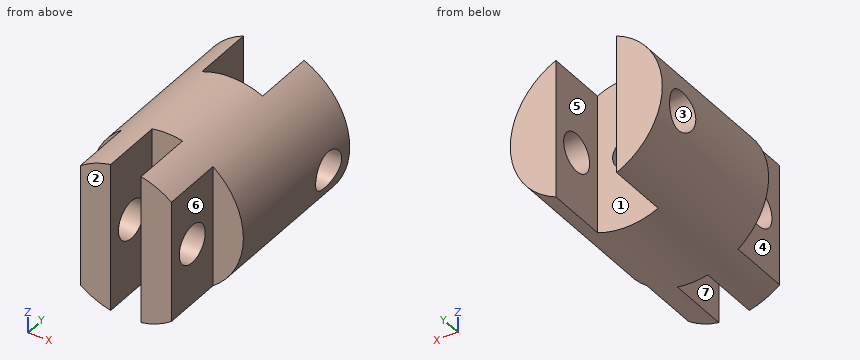
from build123d import *

# Parameters (mm, degrees)
SKETCH1_R               = 12.7
BOSS_EXTRUDE1_DEPTH     = 36.195
CUT_EXTRUDE1_START      = -10.16
CUT_EXTRUDE1_DEPTH      = 10.16
CUT_EXTRUDE2_DEPTH      = 10.16
CUT_EXTRUDE3_DEPTH      = 43.278794034
CUT_EXTRUDE3_DEPTH_BACK = 43.278794034
SKETCH4_R               = 3.175
SKETCH5_R               = 2.54
CUT_EXTRUDE4_DEPTH      = 32.629120053


with BuildPart() as part:
    # Sketch1 → Boss-Extrude1 (new body)
    with BuildSketch(Plane(origin=(0, 0, 0), x_dir=(1, 0, 0), z_dir=(0, 1, 0))):
        with Locations(Location((0, 0, 0), (0, 0, 270))):
            Circle(SKETCH1_R)
    extrude(amount=BOSS_EXTRUDE1_DEPTH)

    # Sketch2 → Cut-Extrude1 (cut)
    with BuildSketch(Plane(origin=(0, 36.195, 0), x_dir=(1, 0, 0), z_dir=(0, 1, 0)).offset(CUT_EXTRUDE1_START)):
        with BuildLine():
            Line((5.08, 11.639742265), (5.08, -11.639742265))
            ThreePointArc((5.08, -11.639742265), (0, -12.7), (-5.08, -11.639742265))
            Line((-5.08, -11.639742265), (-5.08, 11.639742265))
            ThreePointArc((-5.08, 11.639742265), (0, 12.7), (5.08, 11.639742265))
        make_face()
    extrude(amount=CUT_EXTRUDE1_DEPTH, mode=Mode.SUBTRACT)

    # Sketch3 → Cut-Extrude2 (cut)
    with BuildSketch(Plane.XZ):
        with BuildLine():
            Line((-2.54, 12.443407893), (-2.54, -12.443407893))
            ThreePointArc((-2.54, -12.443407893), (0, -12.7), (2.54, -12.443407893))
            Line((2.54, -12.443407893), (2.54, 12.443407893))
            ThreePointArc((2.54, 12.443407893), (0, 12.7), (-2.54, 12.443407893))
        make_face()
        with BuildLine():
            Line((-7.62, 10.16), (-7.62, -10.16))
            ThreePointArc((-7.62, -10.16), (-12.7, 0), (-7.62, 10.16))
        make_face()
        with BuildLine():
            Line((7.62, 10.16), (7.62, -10.16))
            ThreePointArc((7.62, -10.16), (12.7, 0), (7.62, 10.16))
        make_face()
    extrude(amount=-CUT_EXTRUDE2_DEPTH, mode=Mode.SUBTRACT)

    # Sketch4 → Cut-Extrude3 (cut, two sides: drawn at the far end of the back side and taken through both)
    with BuildSketch(Plane(origin=(-5.08, 0, 0), x_dir=(0, 0, -1), z_dir=(1, 0, 0)).offset(-CUT_EXTRUDE3_DEPTH_BACK)):
        with Locations((1.060257735, 31.115)):
            Circle(SKETCH4_R)
        with Locations((0, 5.08)):
            Circle(SKETCH4_R)
    extrude(amount=CUT_EXTRUDE3_DEPTH + CUT_EXTRUDE3_DEPTH_BACK, mode=Mode.SUBTRACT)

    # Sketch5 → Cut-Extrude4 (cut, through all)
    with BuildSketch(Plane(origin=(0, 26.035, 0), x_dir=(1, 0, 0), z_dir=(0, 1, 0))):
        with Locations(Location((0, 0, 0), (0, 0, 270))):
            Circle(SKETCH5_R)
    extrude(amount=-CUT_EXTRUDE4_DEPTH, mode=Mode.SUBTRACT)


solid = part.part
Build history of the part. All positions in model axes, mm. Face numbers are marked on the shaded views. A direction names the side the tool comes from. Round coordinates to 2 decimals unless told otherwise and drop trailing zeros. Write each loop counter-clockwise with the first axis right and the second up, starting at its lowest first coordinate (ties: lowest second). Pieces come first, ordered by that corner, then holes. Notation, with made-up numbers: (56.25, -22.75) -> (70.25, -22.75) arc R31 ccw to (70.25, 2.25) -> close; hole circle Ø2 at (-35, 15.5). An arc over 180 degrees is marked (long way). Write item = value, one per line.
(1) Band-saw the part on D-D (z = -5.25). Give the cut face in (x, y) (3 decimals).
Answer:
outline = (-11.564, 10.16) -> (-7.62, 10.16) -> (-7.62, 0) -> (-2.54, 0) -> (-2.54, 10.16) -> (2.54, 10.16) -> (2.54, 0) -> (7.62, 0) -> (7.62, 10.16) -> (11.564, 10.16) -> (11.564, 36.195) -> (5.08, 36.195) -> (5.08, 26.035) -> (-5.08, 26.035) -> (-5.08, 36.195) -> (-11.564, 36.195) -> close
(2) Band-saw the part on B-B (x = 0). Give the cut face in (y, z) (3 decimals), then the cut area to 3 significant figures.
Answer:
outline = (10.16, -12.7) -> (26.035, -12.7) -> (26.035, -2.54) -> (10.16, -2.54) -> close; (10.16, 2.54) -> (26.035, 2.54) -> (26.035, 12.7) -> (10.16, 12.7) -> close
area = 323 mm2
(3) Tool access for the marked faces 4, 5, 6 and 7: list every direction of +Z, -Z, +X, -X, +Y, -Y with a clear straight run to the whole face (end or side of a thin tool).
Answer:
face_4 = +Z, -Z, -X, -Y
face_5 = +Z, -Z, +Y
face_6 = +Z, -Z, +X, -Y
face_7 = +Z, -Z, -Y
(4) Probe L1, parallel to X at y = 18.5, z = 0; L2, parallel to X at y = 3, z = 9. List the from-to ranges inside material, lowest first.
Answer:
L1 = -12.7 to -2.54, 2.54 to 12.7
L2 = -7.62 to -2.54, 2.54 to 7.62
(5) Two-plate mould, pull along Y, no slides. Class the marked faces 1, 2 and 3: pulls with the +Y half, pulls with the -Y half, needs draft (parallel to the pull), parting line crosses it, or undercut.
Answer:
face_1 = pulls with the +Y half
face_2 = pulls with the -Y half
face_3 = undercut
(6) Flat gauge pins, fed straight in: pin 1 (8 mm diameter, centred on y = 3.5, z = 3.5, fed in from +X); pin 2 (10 mm diameter, centred on x = 0.5, z = -5.5, fed in from +Y) (3 decimals); pin 3 (5 mm diameter, centred on x = -9.5, y = 19, fed in from +Z); pin 4 (1.5 mm diameter, centred on x = 10, z = 1, fed in from -Y). Where does each tip first touch, or does it go through?
Answer:
pin_1 = 7.62
pin_2 = 36.195
pin_3 = 10.6
pin_4 = 10.16
(7) Band-saw the part on A-A (y = 5.08). Give the cut face in (x, z) (3 decimals), then the cut area to 3 significant figures.
Answer:
outline = (-7.62, -10.16) arc R12.7 ccw to (-2.54, -12.443) -> (-2.54, -3.175) -> (-7.62, -3.175) -> close; (-7.62, 3.175) -> (-2.54, 3.175) -> (-2.54, 12.443) arc R12.7 ccw to (-7.62, 10.16) -> close; (2.54, -12.443) arc R12.7 ccw to (7.62, -10.16) -> (7.62, -3.175) -> (2.54, -3.175) -> close; (2.54, 3.175) -> (7.62, 3.175) -> (7.62, 10.16) arc R12.7 ccw to (2.54, 12.443) -> close
area = 170 mm2
(8) Band-saw the part on C-C (x = 4.25). Give the cut face in (y, z) (3 decimals), then the cut area to 3 significant figures.
Answer:
outline = (0, -11.968) -> (26.035, -11.968) -> (26.035, 11.968) -> (0, 11.968) -> close; hole circle Ø6.35 at (5.08, 0)
area = 591 mm2
